Answer from the drawing. Dimensions are ordinates in mm from the lowest x, y and z of the part. A direction names the side the tool comes from. Coordinates: 2 decimals unless noted, no trailing zeros. Order: outer loops, then holes, each group sorted by start corner. A loop starts at its lowest first (then second) coordinate and runs counter-clockwise, first axis right, second up. Notation, with made-up numbers: (88.5, 39.25) - (121.5, 39.25) arc R7 ccw to (121.5, 50.25) - close; hole circle Ø8 at (-34, -21.5). An arc over 180 degrees is marked (long way). One line per item, written item: value. Start each with the question number.
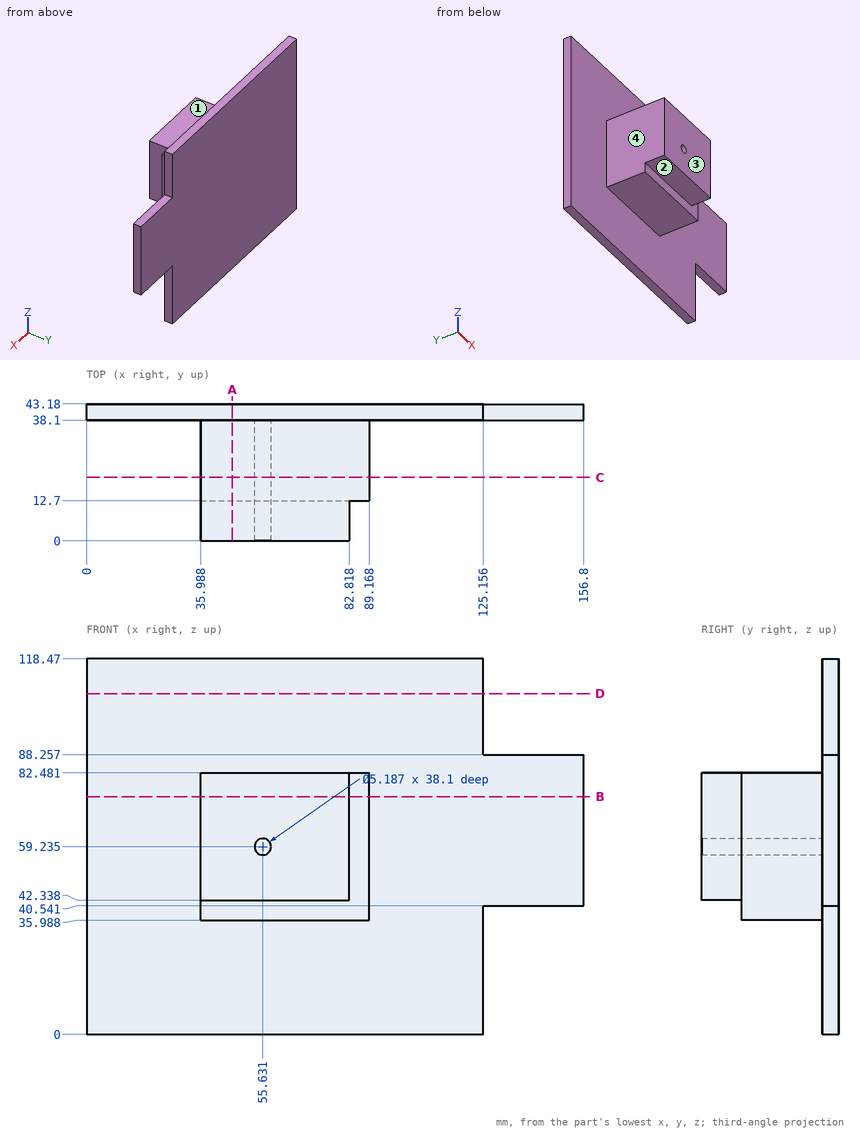
(1) The part is cut by section C-C on y = 20. Determine the outline of the cut face in (x, z) (1 decimal).
(2) Flat-ended cylindrical pins translate along their axes: pin 1 Ø1.6 at (x, z) = (56, 59.5) entering from -Y; pin 2 Ø2 at (y, z) = (15, 37) entering from +X; pin 3 Ø10 at (y, z) = (4, 54) entering from +X; pin 4 Ø23 at (x, z) = (72, 70.5) entering from -Y. Find the tip coordinate at first contact, or state that the pin passes through.
(3) The part is cut by section D-D on z = 107.5. Determine the outline of the cut face in (x, y).
(4) For the marked faces 1, 2, 3 and 4, determine the directions among +Z, -Z, +X, -X, +Y, -Y from which every point of the face is accessible in a straight line to the end or side of a thin tool.
(5) Consider probe 1 along Y at (x, z) = (28.5, 87); probe 2 along X at (y, z) = (20, 73.5); probe 3 along Z at (x, y) = (64, 5). Determine where each line is inside the solid, lowest interval first.
(6) The part is cut by section B-B on z = 75. Determine the outline of the cut face in (x, y).
(7) The part is cut by section A-A on x = 46. Determine the outline of the cut face in (y, z).
Completed:
1. outline: (36, 36) - (89.2, 36) - (89.2, 82.5) - (36, 82.5) - close; hole circle Ø5.2 at (55.6, 59.2)
2. pin 1: stops at y = 38.1
2. pin 2: stops at x = 89.17
2. pin 3: stops at x = 82.82
2. pin 4: stops at y = 0
3. outline: (0, 38.1) - (125.16, 38.1) - (125.16, 43.18) - (0, 43.18) - close
4. face 1: +Z, +X, -X, -Y
4. face 2: -Z, +X, -X, -Y
4. face 3: +Z, -Z, +X, -X, -Y
4. face 4: +Z, -Z, -X, -Y
5. probe 1: y = 38.1 to 43.18
5. probe 2: x = 35.99 to 89.17
5. probe 3: z = 42.34 to 82.48
6. outline: (0, 38.1) - (35.99, 38.1) - (35.99, 0) - (82.82, 0) - (82.82, 12.7) - (89.17, 12.7) - (89.17, 38.1) - (156.8, 38.1) - (156.8, 43.18) - (0, 43.18) - close
7. outline: (0, 42.34) - (12.7, 42.34) - (12.7, 35.99) - (38.1, 35.99) - (38.1, 0) - (43.18, 0) - (43.18, 118.47) - (38.1, 118.47) - (38.1, 82.48) - (0, 82.48) - close
